from build123d import *

# Parameters (mm, degrees)
SKETCH1_R               = 35
BOSS_EXTRUDE1_DEPTH     = 60
CUT_EXTRUDE2_DEPTH      = 212.187120971
CUT_EXTRUDE2_DEPTH_BACK = 212.187120971
SKETCH3_OUTSIDE_W       = 299.272
SKETCH3_OUTSIDE_H       = 179.272
SKETCH3_OUTSIDE_R       = 35


with BuildPart() as part:
    # Sketch1 → Boss-Extrude1 (new, symmetric)
    with BuildSketch(Plane(origin=(0, 0, 0), x_dir=(1, 0, 0), z_dir=(0, 1, 0))):
        with BuildLine():
            Line((90, 20), (190, 20))
            Line((190, 20), (190, -20))
            Line((190, -20), (90, -20))
            add(Edge.make_bspline(
                [(30, -40), (53.522105639, -22.358420771), (73.740829121, -19.957299765), (90, -20)],
                knots=[0, 0, 0, 0, 0.5, 0.5, 0.5, 0.5], degree=3))
            ThreePointArc((30, -40), (-50, 0), (30, 40))
            add(Edge.make_bspline(
                [(30, 40), (53.522105639, 22.358420771), (73.740829121, 19.957299765), (90, 20)],
                knots=[0, 0, 0, 0, 0.5, 0.5, 0.5, 0.5], degree=3))
        make_face()
        with Locations(Location((0, 0, 0), (0, 0, 270))):
            Circle(SKETCH1_R, mode=Mode.SUBTRACT)
    extrude(amount=BOSS_EXTRUDE1_DEPTH, both=True)

    # Sketch3 outside → Cut-Extrude2 (cut, two sides: drawn at the far end of the back side and taken through both)
    # profile 1 of 2: a face of its own
    with BuildSketch(Plane(origin=(0, 0, -20), x_dir=(-1, 0, 0), z_dir=(0, 0, -1)).offset(-CUT_EXTRUDE2_DEPTH_BACK)):
        with Locations((-70, 0)):
            Rectangle(SKETCH3_OUTSIDE_W, SKETCH3_OUTSIDE_H)
        with BuildLine():
            Line((-50, -20), (50, -20))
            Line((50, -20), (50, 20))
            Line((50, 20), (-50, 20))
            add(Edge.make_bspline(
                [(-110, 40), (-99.496724582, 32.122543436), (-87.389560029, 27.685973517), (-61.506465559, 20), (-50, 20)],
                knots=[0, 0, 0, 0, 0.549428734, 1, 1, 1, 1], degree=3))
            ThreePointArc((-110, 40), (-190, 0), (-110, -40))
            add(Edge.make_bspline(
                [(-110, -40), (-100.093364528, -32.570023396), (-80.659161516, -23.139318123), (-60.932096988, -20), (-50, -20)],
                knots=[0, 0, 0, 0, 0.546701071, 1, 1, 1, 1], degree=3))
        make_face(mode=Mode.SUBTRACT)
    # profile 2 of 2: a face of its own
    with BuildSketch(Plane(origin=(0, 0, -20), x_dir=(-1, 0, 0), z_dir=(0, 0, -1)).offset(-CUT_EXTRUDE2_DEPTH_BACK)):
        with Locations((-140, 0)):
            Circle(SKETCH3_OUTSIDE_R)
    extrude(amount=CUT_EXTRUDE2_DEPTH + CUT_EXTRUDE2_DEPTH_BACK, mode=Mode.SUBTRACT)


solid = part.part
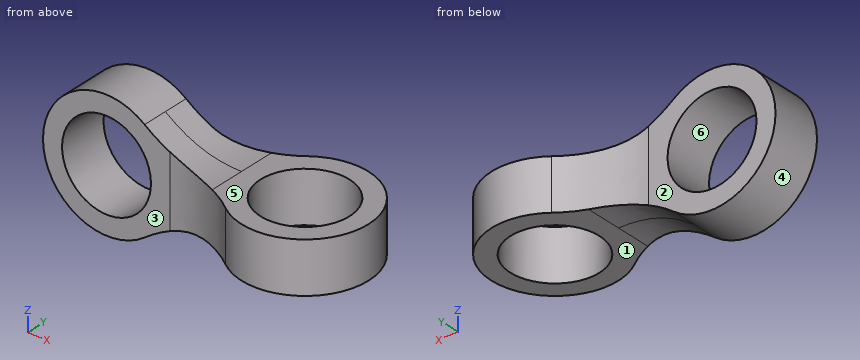
Verification items for the finished model (mm, model axes). Face numbers are marked on the shaded views. A direction names the side the tool comes from. Give positions to 0.01 mm unless a question says otherwise; leave off trailing zeros. Loops run counter-clockwise (first coordinate to the right, second up) from the corner with the lowest first, then second, coordinate; pieces in that order, holes last. Notation, with made-up numbers: (74, 25) - (105, 25) arc R26 ccw to (105, 55) - close; hole circle Ø4 at (29.25, 6.25). An arc over 180 degrees is marked (long way). Write each question's results on one line, items separated by ' | '.
1) Sectioned sample at A-A on x = 140. Record the boundary of the cut face in (y, z), plus the area to 3 significant figures.
Solution:
outline: (-50, -20) - (-35, -20) - (-35, 20) - (-50, 20) - close; (35, -20) - (50, -20) - (50, 20) - (35, 20) - close | area: 1,200 mm2
2) Material ranges on L1, parallel to Z at x = 0, y = 7; L2, parallel to X at y = -18, z = -1, recorded low to high. Write a range as from..to.
Solution:
L1: -50..-35, 35..50 | L2: -49.99..-34.99, 34.99..109.98, 170.02..186.65
3) Mould release check, pull along Z, two halves, no side actions. Record for the marked faces 4, 5 and 6: pulls with the +Z half, pulls with the -Z half, needs draft (parallel to the pull), parting line crosses it, or undercut.
Solution:
face 4: parting line crosses it | face 5: pulls with the +Z half | face 6: undercut
4) Sectioned sample at D-D on x = -21. Record the boundary of the cut face in (y, z), plus the area to 3 significant figures.
Solution:
outline: (-20, -45.38) - (20, -45.38) - (20, -28) - (-20, -28) - close; (-20, 28) - (20, 28) - (20, 45.38) - (-20, 45.38) - close | area: 1,390 mm2
5) Sectioned sample at B-B on z = 0. Count the separate pieces of the cut face and the enclosed holes in it, plus the area to 3 significant figures.
Solution:
separate pieces: 2 | enclosed holes: 1 | area: 7,280 mm2
6) Tool access check on the marked faces 1, 2 and 3. Record the directions out of +Z, -Z, +X, -X, +Y, -Y that give a thin tool (end or side, any length) a straight path to the whole face; none if there is none.
Solution:
face 1: -Z, +X, +Y, -Y | face 2: +Z, -Z, -X, +Y | face 3: +Z, -Z, -X, -Y
7) Depth check by flat-ended pin: P1, Ø1, axis at x = 119.5, z = 11, coming from the +Y side; P2, Ø12, axis at x = 87.5, y = -18.5, coming from the -Z side; P3, Ø2, axis at x = 42, z = -2, coming from the +Y side. Enter the tip coordinate at first touch or a pass-through.
Solution:
P1: y = 45.83 | P2: z = -20.24 | P3: y = 20
